Can you work these out from the model? Positions are in its coordinate system, mm. Round coordinates to 2 decimals unless told otherwise and drop trailing zeros. Write each loop counter-clockwise with the first axis right and the second up, starting at its lowest first coordinate (ties: lowest second). Pieces come first, ordered by that corner, then holes. Notation, with made-up numbers: (77.5, 33) -> (108.5, 33) arc R15 cw to (108.5, 58) -> close; hole circle Ø5 at (27.25, 48). An arc over 180 degrees is marked (long way). Use CSV: the item, a comma, the result in double quotes.
```python
from build123d import *

# Parameters (mm, degrees)
F0_R          = 20.4
F0_R_2        = 18.9
F1_DEPTH      = 4
F0_R_3        = 2.5
F0_R_4        = 8
F2_DEPTH      = 4
F3_DEPTH      = 4
F4_R          = 5
F4_R_2        = 2.5
F5_DEPTH      = 6
F4_R_3        = 1.5
F6_DEPTH      = 6
F4_R_4        = 8
F4_R_5        = 6
F7_DEPTH      = 5
F7_DEPTH_BACK = 1
F8_R          = 5
F9_D          = 5
F4_R_6        = 6.7492124295
F4_R_7        = 8.8034997794
F4_R_8        = 7.7469148922
F10_DEPTH     = 6.001


with BuildPart() as f1:
    # F0 (on Top) → F1 (new body)
    with BuildSketch(Plane.XY):
        Circle(F0_R)
        Circle(F0_R_2, mode=Mode.SUBTRACT)
    extrude(amount=-F1_DEPTH)

    # F0 (on Top) → F2 (join)
    with BuildSketch(Plane.XY):
        with BuildLine():
            Line((-37.9369594157, 71.9021782279), (-73.2717439532, -15.7500002533))
            Line((-73.2717439532, -15.7500002533), (-33.7380266771, -31.6870300696))
            Line((-33.7380266771, -31.6870300696), (0, -23.96739088))
            ThreePointArc((0, -23.96739088), (14.4587631047, -16.2687135057), (23.0604634443, -2.3282610346))
            Line((23.0604634443, -2.3282610346), (23.0604634443, 47.3125920767))
            Line((23.0604634443, 47.3125920767), (-37.9369594157, 71.9021782279))
        make_face()
        with Locations((-30.9, 0)):
            Circle(F0_R_3, mode=Mode.SUBTRACT)
        Circle(F0_R, mode=Mode.SUBTRACT)
        with Locations((-19.5403950401, 28.736203214)):
            Circle(F0_R_4, mode=Mode.SUBTRACT)
    extrude(amount=-F2_DEPTH)

    # F0 (on Top) → F3 (join)
    with BuildSketch(Plane.XY):
        Circle(F0_R_2)
    extrude(amount=-F3_DEPTH)

    # F4 (on face) → F5 (join)
    with BuildSketch(Plane.XY):
        with Locations((-30.8152195066, 0)):
            Circle(F4_R)
        with Locations((-30.9, 0)):
            Circle(F4_R_2, mode=Mode.SUBTRACT)
    extrude(amount=-F5_DEPTH)

    # F4 (on face) → F6 (join)
    with BuildSketch(Plane.XY):
        with Locations((15.0604634443, 36.3125920767)):
            Circle(F4_R)
        with Locations((15.0604634443, 36.3125920767)):
            Circle(F4_R_3, mode=Mode.SUBTRACT)
        with Locations((-33.5082715717, 61.4912837428)):
            Circle(F4_R)
        with Locations((-33.5082715717, 61.4912837428)):
            Circle(F4_R_3, mode=Mode.SUBTRACT)
        with Locations((-62.8608494681, -11.3213124094)):
            Circle(F4_R)
        with Locations((-62.8608494681, -11.3213124094)):
            Circle(F4_R_3, mode=Mode.SUBTRACT)
    extrude(amount=-F6_DEPTH)

    # F4 (on face) → F7 (join, two sides)
    with BuildSketch(Plane.XY) as f7_sk:
        with Locations((-19.5403950401, 28.736203214)):
            Circle(F4_R_4)
        with Locations((-19.5659566671, 28.7475492805)):
            Circle(F4_R_5, mode=Mode.SUBTRACT)
    extrude(amount=-F7_DEPTH)
    extrude(f7_sk.sketch, amount=F7_DEPTH_BACK)

    # F8
    f8_edges = [f1.edges().sort_by_distance(p)[0] for p in [
        (-73.271744, -15.75, -2),
        (-37.936959, 71.902178, -2),
        (23.060463, 47.312592, -2),
        (-33.738027, -31.68703, -2),
    ]]
    fillet(f8_edges, radius=F8_R)

    # F9 (through all)
    with Locations(Plane.XY):
        with Locations((-33.5082715717, 61.4912837428), (15.0604634443, 36.3125920767), (-62.8608494681, -11.3213124094)):
            Hole(F9_D / 2)

    # F4 (on face) → F10 (cut, through all)
    with BuildSketch(Plane.XY):
        with Locations((-24.8405560851, 46.2679713964)):
            Circle(F4_R_6)
        with BuildLine():
            ThreePointArc((-34.5543373603, 32.8433099638), (-39.1188131875, 36.5180985692), (-44.0384065292, 33.3343724152))
            Line((-44.0384065292, 33.3343724152), (-52.4302117947, 11.7191193495))
            ThreePointArc((-52.4302117947, 11.7191193495), (-51.444320935, 6.5193730929), (-46.340876706, 5.1178742801))
            Line((-46.340876706, 5.1178742801), (-33.1174276827, 9.0594797734))
            ThreePointArc((-33.1174276827, 9.0594797734), (-30.1749819218, 11.422822336), (-29.7226936025, 15.1696623914))
            Line((-29.7226936025, 15.1696623914), (-34.5543373603, 32.8433099638))
        make_face()
        with BuildLine():
            Line((5.2675922587, 22.2754651912), (-4.5154558015, 20.7042452523))
            ThreePointArc((-4.5154558015, 20.7042452523), (-6.2156561453, 20.1016297559), (-7.5913755862, 18.9349152813))
            ThreePointArc((-7.5913755862, 18.9349152813), (1.9526532516, 20.3063326398), (11.0604634443, 17.1413578341))
            Line((11.0604634443, 17.1413578341), (11.0604634443, 17.3387299053))
            ThreePointArc((11.0604634443, 17.3387299053), (9.3035826274, 21.1442755907), (5.2675922587, 22.2754651912))
        make_face()
        with BuildLine():
            ThreePointArc((11.0604634443, 17.1413578341), (1.9526532516, 20.3063326398), (-7.5913755862, 18.9349152813))
            ThreePointArc((-7.5913755862, 18.9349152813), (-7.7960820291, 18.6669269466), (-7.9822585437, 18.3857494569))
            Line((-7.9822585437, 18.3857494569), (-20.3289314836, -1.7013361619))
            ThreePointArc((-20.3289314836, -1.7013361619), (-18.3724422175, -8.866417933), (-13.9804985925, -14.8561656932))
            Line((-13.9804985925, -14.8561656932), (-6.7808091525, -13.2087959378))
            ThreePointArc((-6.7808091525, -13.2087959378), (3.5211433289, -8.4701576249), (11.0604634443, 0))
            Line((11.0604634443, 0), (11.0604634443, 17.1413578341))
        make_face()
        with BuildLine():
            ThreePointArc((-13.9804985925, -14.8561656932), (-18.3724422175, -8.866417933), (-20.3289314836, -1.7013361619))
            Line((-20.3289314836, -1.7013361619), (-24.5383981985, -8.5498141869))
            ThreePointArc((-24.5383981985, -8.5498141869), (-24.341412043, -14.0825979067), (-19.1634895492, -16.0420921996))
            Line((-19.1634895492, -16.0420921996), (-13.9804985925, -14.8561656932))
        make_face()
        with Locations((-41.2170253694, -13.2419364527)):
            Circle(F4_R_7)
        with Locations((-3.5378288012, 42.4071475863)):
            Circle(F4_R_8)
    extrude(amount=-F10_DEPTH, mode=Mode.SUBTRACT)


solid = f1.part
```
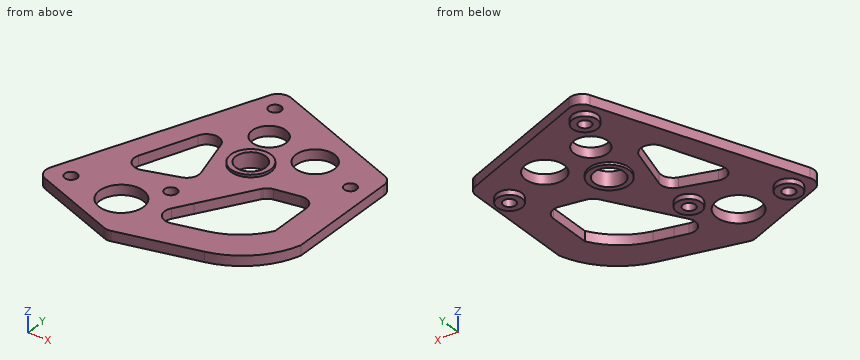
Q1. Will these pins go through, and if not, where does the flat tip stop? P1, Ø2, axis at y = 13, z = -2.5, coming from the -X side (3 decimals); P2, Ø4, axis at x = -15, y = -15, coming from the +Z side; P3, Ø8, axis at x = -16.5, y = 31.5, coming from the -Z side; P4, Ø8, axis at x = -33.51, y = 61.49, coming from the -Z side.
Resolved:
P1,"stops at x = -62.085"
P2,"stops at z = 0"
P3,"stops at z = -5"
P4,"stops at z = -6"
Q2. Please list where these lines run through material, in increasing order: probe 1 along X at (y, z) = (15, -0.75); probe 2 along X at (y, z) = (41.5, -2.75); probe 3 along Y at (x, z) = (-63, -0.5).
Resolved:
probe 1,"x = -60.88 to -51.16, -29.68 to -10.06, 11.06 to 23.06"
probe 2,"x = -50.19 to -29.62, -20.06 to -11.23, 4.16 to 23.06"
probe 3,"y = -19.89 to -13.82, -8.83 to 9.73"
Q3. Suppose I cut it at B-B (y = 26). Write out the boundary of the cut face in (x, z), and give its area (3 significant figures).
Resolved:
outline,"(-56.44, -4) -> (-46.89, -4) -> (-46.89, 0) -> (-56.44, 0) -> close; (-32.68, -4) -> (-27.06, -4) -> (-27.06, -5) -> (-24.9, -5) -> (-24.9, 1) -> (-27.06, 1) -> (-27.06, 0) -> (-32.68, 0) -> close; (-14.23, -5) -> (-12.02, -5) -> (-12.02, -4) -> (23.06, -4) -> (23.06, 0) -> (-12.02, 0) -> (-12.02, 1) -> (-14.23, 1) -> close"
area,"227 mm^2"
Q4. Suppose I cut it at A-A (x = -1.5). Write out the boundary of the cut face in (y, z).
Resolved:
outline,"(-24.31, -4) -> (-11.43, -4) -> (-11.43, 0) -> (-24.31, 0) -> close; (21.19, -4) -> (34.93, -4) -> (34.93, 0) -> (21.19, 0) -> close; (49.88, -4) -> (57.21, -4) -> (57.21, 0) -> (49.88, 0) -> close"
